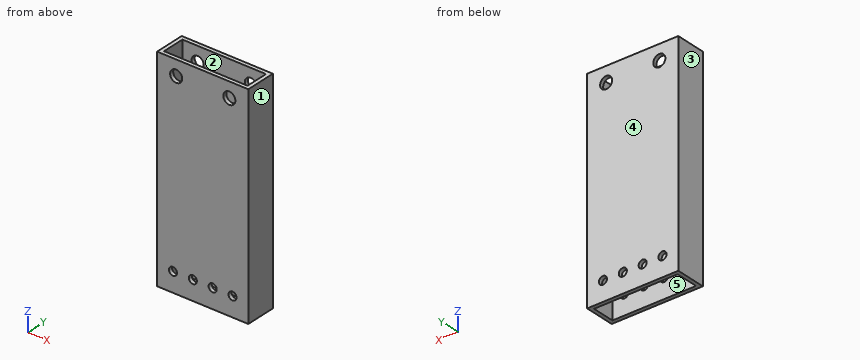
```python
from build123d import *

# Parameters (mm, degrees)
SKETCH1_W           = 76.2
SKETCH1_H           = 25.4
SKETCH1_W_2         = 69.85
SKETCH1_H_2         = 19.05
BOSS_EXTRUDE1_DEPTH = 177.8
SKETCH4_R           = 3.3782
CUT_EXTRUDE1_DEPTH  = 26.4
SKETCH5_R           = 5.0419
CUT_EXTRUDE2_DEPTH  = 26.4


with BuildPart() as part:
    # Sketch1 → Boss-Extrude1 (new body)
    with BuildSketch(Plane.XY):
        with Locations((38.1, 12.7)):
            Rectangle(SKETCH1_W, SKETCH1_H)
        with Locations((38.1, 12.7)):
            Rectangle(SKETCH1_W_2, SKETCH1_H_2, mode=Mode.SUBTRACT)
    extrude(amount=BOSS_EXTRUDE1_DEPTH)

    # Sketch4 → Cut-Extrude1 (cut, through all)
    with BuildSketch(Plane(origin=(0, 25.4, 0), x_dir=(1, 0, 0), z_dir=(0, 1, 0))):
        with Locations((13.21308, -16.2687)):
            Circle(SKETCH4_R)
        with Locations((29.80436, -16.2687)):
            Circle(SKETCH4_R)
        with Locations((46.39564, -16.2687)):
            Circle(SKETCH4_R)
        with Locations((62.98692, -16.2687)):
            Circle(SKETCH4_R)
    extrude(amount=-CUT_EXTRUDE1_DEPTH, mode=Mode.SUBTRACT)

    # Sketch5 → Cut-Extrude2 (cut, through all)
    with BuildSketch(Plane.XZ):
        with Locations((60.325, 165.1)):
            Circle(SKETCH5_R)
        with Locations((15.875, 165.1)):
            Circle(SKETCH5_R)
    extrude(amount=-CUT_EXTRUDE2_DEPTH, mode=Mode.SUBTRACT)


solid = part.part
```
Geometry: final body of the model. Coordinates: model frame, mm. Face numbers are marked on the shaded views. A direction names the side the tool comes from. Round coordinates to 2 decimals unless told otherwise and drop trailing zeros. Write each loop counter-clockwise with the first axis right and the second up, starting at its lowest first coordinate (ties: lowest second). Pieces come first, ordered by that corner, then holes. Notation, with made-up numbers: (58.25, 76) -> (111.25, 76) arc R20 ccw to (111.25, 110) -> close; hole circle Ø8 at (76, 39). An arc over 180 degrees is marked (long way). Return JSON: item names as keys, results as strings.
Q1. Section B-B on y = 9.5. Return the cut outline in (x, z) (3 decimals), and give its area (3 significant figures).
From the geometry:
{"outline": "(0, 0) -> (3.175, 0) -> (3.175, 177.8) -> (0, 177.8) -> close; (73.025, 0) -> (76.2, 0) -> (76.2, 177.8) -> (73.025, 177.8) -> close", "area": "1,130 mm2"}
Q2. Section A-A on z = 165.1. Return the cut outline in (x, y) (3 decimals).
From the geometry:
{"outline": "(0, 0) -> (10.833, 0) -> (10.833, 3.175) -> (3.175, 3.175) -> (3.175, 22.225) -> (10.833, 22.225) -> (10.833, 25.4) -> (0, 25.4) -> close; (20.917, 0) -> (55.283, 0) -> (55.283, 3.175) -> (20.917, 3.175) -> close; (20.917, 22.225) -> (55.283, 22.225) -> (55.283, 25.4) -> (20.917, 25.4) -> close; (65.367, 0) -> (76.2, 0) -> (76.2, 25.4) -> (65.367, 25.4) -> (65.367, 22.225) -> (73.025, 22.225) -> (73.025, 3.175) -> (65.367, 3.175) -> close"}
Q3. First-contact query: pin 1 Ø4 at (x, z) = (13.21, 16.27) entering from +Y. Flat tip, straight axial feed; report the tip coordinate or a pass-through.
From the geometry:
{"pin 1": "through"}
Q4. Section C-C on x = 70. Return the cut outline in (y, z) (3 decimals).
From the geometry:
{"outline": "(0, 0) -> (3.175, 0) -> (3.175, 177.8) -> (0, 177.8) -> close; (22.225, 0) -> (25.4, 0) -> (25.4, 177.8) -> (22.225, 177.8) -> close"}
Q5. Section D-D on z = 86. Return the cut outline in (x, y) (3 decimals).
From the geometry:
{"outline": "(0, 0) -> (76.2, 0) -> (76.2, 25.4) -> (0, 25.4) -> close; hole (3.175, 3.175) -> (73.025, 3.175) -> (73.025, 22.225) -> (3.175, 22.225) -> close"}
Q6. Mould query, pull axis X, two halves, no side actions, for the marked faces 3, 4 and 5. Classes: +X half, -X half, draft (parallel to the pull), parting line (faces both ways), or undercut.
From the geometry:
{"face 3": "-X half", "face 4": "draft", "face 5": "undercut"}
Q7. Ray query, line 1 (X direction, y = 6, z = 141.5) (3 decimals); line 2 (Y direction, x = 70, z = 159.5) (3 decimals); line 3 (Z direction, x = 14, y = 2.5). Return the intervals inside material, ascending.
From the geometry:
{"line 1": "0 to 3.175, 73.025 to 76.2", "line 2": "0 to 3.175, 22.225 to 25.4", "line 3": "0 to 12.98, 19.55 to 160.42, 169.78 to 177.8"}
Q8. Set-up query: the marked faces 1 and 2. Return all of +Z, -Z, +X, -X, +Y, -Y with unobstructed straight access to the full face (end or side cutting, diameter ignored); none if empty.
From the geometry:
{"face 1": "+Z, -Z, +X, +Y, -Y", "face 2": "+Z, -Z"}
